Could you check a few things on this model? Use its own coordinates, in mm. Face numbers are marked on the shaded views. A direction names the side the tool comes from. Give positions to 0.01 mm unless a question says otherwise; leave off trailing zeros. Order: outer loops, then holes, each group sorted by start corner. A loop starts at its lowest first (then second) coordinate and runs counter-clockwise, first axis right, second up. Notation, with made-up numbers: (-22, 66) -> (-16, 66) arc R23 ccw to (-16, 99) -> close; hole circle Ø6 at (-36.5, 49). An arc over 180 degrees is marked (long way). Use one line per item in the form item = value. Start each with the question number.
from build123d import *

# Parameters (mm, degrees)
BOSS_EXTRUDE1_DEPTH          = 29
CUT_EXTRUDE1_DEPTH           = 96.799008346
CUT_EXTRUDE2_DEPTH           = 96.799008346
CUT_EXTRUDE2_DEPTH_BACK      = 96.799008346
SKETCH4_W                    = 32.25
SKETCH4_H                    = 6
SKETCH5_W                    = 175.4
SKETCH5_H                    = 34
CUT_EXTRUDE3_DEPTH           = 20.4
SKETCH6_W                    = 29.649504938
SKETCH6_H                    = 34
CUT_EXTRUDE4_DEPTH           = 95.596247283
SKETCH7_W                    = 29.649504938
SKETCH7_H                    = 34
CUT_EXTRUDE5_DEPTH           = 95.596247283
F_5_32_0_14_DIAMETER_HOLE1_D = 3.556
SKETCH13_R                   = 4
CUT_EXTRUDE6_DEPTH           = 106.908356611
FILLET1_R                    = 10
FILLET2_R                    = 10


with BuildPart() as part:
    # Sketch1 → Boss-Extrude1 (new, symmetric)
    with BuildSketch(Plane(origin=(0, 0, 0), x_dir=(1, 0, 0), z_dir=(0, 1, 0))):
        with BuildLine():
            Line((-12.7, 75), (-12.7, -75))
            ThreePointArc((-12.7, -75), (0, -87.7), (12.7, -75))
            Line((12.7, -75), (12.7, 75))
            ThreePointArc((12.7, 75), (0, 87.7), (-12.7, 75))
        make_face()
    extrude(amount=BOSS_EXTRUDE1_DEPTH, both=True)

    # Sketch3 → Cut-Extrude1 (cut, symmetric)
    with BuildSketch(Plane.ZY.offset(12.7)):
        Polygon((-45, 29), (-32.009618943, 21.5), (32.009618943, 21.5), (45, 29), align=None)
    cut_extrude1 = extrude(amount=CUT_EXTRUDE1_DEPTH, both=True, mode=Mode.SUBTRACT)

    # Mirror1: Cut-Extrude1 across plane
    add(cut_extrude1.mirror(Plane.ZX), mode=Mode.SUBTRACT)

    # Sketch4 → Cut-Extrude2 (cut, two sides: drawn at the far end of the back side and taken through both)
    with BuildSketch(Plane.ZY.offset(12.7).offset(-CUT_EXTRUDE2_DEPTH_BACK)):
        with Locations((71.575, 20)):
            Rectangle(SKETCH4_W, SKETCH4_H)
        with Locations((-71.575, 20)):
            Rectangle(SKETCH4_W, SKETCH4_H)
        with Locations((-71.575, -20)):
            Rectangle(SKETCH4_W, SKETCH4_H)
        with Locations((71.575, -20)):
            Rectangle(SKETCH4_W, SKETCH4_H)
    extrude(amount=CUT_EXTRUDE2_DEPTH + CUT_EXTRUDE2_DEPTH_BACK, mode=Mode.SUBTRACT)

    # Sketch5 → Cut-Extrude3 (cut)
    with BuildSketch(Plane.ZY.offset(12.7)):
        Rectangle(SKETCH5_W, SKETCH5_H)
    extrude(amount=-CUT_EXTRUDE3_DEPTH, mode=Mode.SUBTRACT)

    # Sketch6 → Cut-Extrude4 (cut, through all)
    with BuildSketch(Plane.ZY.offset(-7.7)):
        with Locations((70.274752469, 0)):
            Rectangle(SKETCH6_W, SKETCH6_H)
    extrude(amount=-CUT_EXTRUDE4_DEPTH, mode=Mode.SUBTRACT)

    # Sketch7 → Cut-Extrude5 (cut, through all)
    with BuildSketch(Plane.ZY.offset(-7.7)):
        with Locations((-70.274752469, 0)):
            Rectangle(SKETCH7_W, SKETCH7_H)
    extrude(amount=-CUT_EXTRUDE5_DEPTH, mode=Mode.SUBTRACT)

    # 5/32 (0.14) Diameter Hole1 (through all)
    with Locations(Plane(origin=(0, 29, 0), x_dir=(1, 0, 0), z_dir=(0, 1, 0))):
        with Locations((0, -65.221), (-9.779, -75), (9.779, -75), (0, -84.779)):
            f_5_32_0_14_diameter_hole1 = Hole(F_5_32_0_14_DIAMETER_HOLE1_D / 2)

    # Mirror3: 5/32 (0.14) Diameter Hole1 across plane
    add(f_5_32_0_14_diameter_hole1.mirror(Plane.XY), mode=Mode.SUBTRACT)

    # Sketch13 → Cut-Extrude6 (cut, symmetric)
    with BuildSketch(Plane.XZ.offset(29)):
        with Locations(Location((0, -75, 0), (0, 0, 270))):
            Circle(SKETCH13_R)
    cut_extrude6 = extrude(amount=CUT_EXTRUDE6_DEPTH, both=True, mode=Mode.SUBTRACT)

    # Mirror4: Cut-Extrude6 across plane
    add(cut_extrude6.mirror(Plane.XY), mode=Mode.SUBTRACT)

    # Fillet1
    fillet1_edges = [part.edges().sort_by_distance(p)[0] for p in [
        (7.7, 17, 0),
    ]]
    fillet(fillet1_edges, radius=FILLET1_R)

    # Fillet2
    fillet2_edges = [part.edges().sort_by_distance(p)[0] for p in [
        (7.7, -17, 0),
    ]]
    fillet(fillet2_edges, radius=FILLET2_R)


solid = part.part
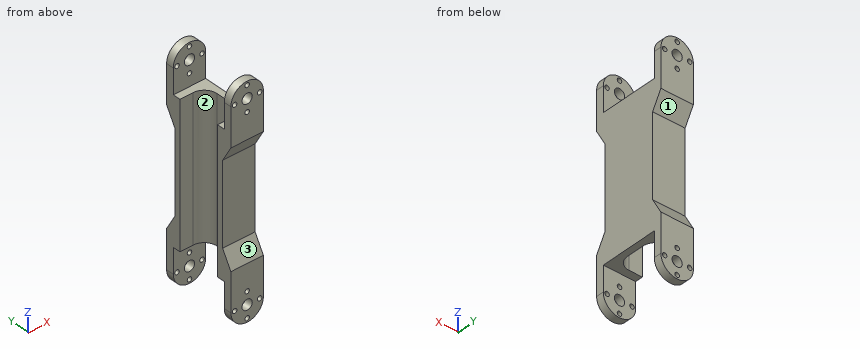
(1) I'm going to push flat-ended pins straight in: pin 1 Ø3 at (x, z) = (0, -65.221) entering from -Y; pin 2 Ø1 at (x, y) = (8, 6) entering from +Z; pin 3 Ø5 at (x, z) = (-5, 32.5) entering from -Y; pin 4 Ø8.5 at (x, z) = (-5, -13.5) entering from +Y. Where does each tip first touch, or does it pass through?
(2) Imagine slicing it at B-B (y = -3.5). Write out the boundary of the cut face in (x, z).
(3) Please list where these lines run through material, in increasing order: probe 1 along X at (y, z) = (-24, 75); probe 2 along Y at (x, z) = (-8.5, -60); probe 3 along Z at (x, y) = (2.5, 25.5).
(4) Imagine slicing it at C-C (z = 29). Write out the boundary of the cut face in (x, y), plus the area to 3 significant figures.
(5) Which directions (+Z, -Z, +X, -X, +Y, -Y) give clear straight access to the entire face, cutting with the end or side of a thin tool? Please do the marked faces 1, 2 and 3.
(6) Imagine slicing it at A-A (z = 47.5). Write out the boundary of the cut face in (x, y).
(7) Imagine slicing it at D-D (x = 10). Give the number of separate pieces and of enclosed holes in the cut face, plus the area to 3 significant figures.
Calculated:
q1.pin_1 = through
q1.pin_2 = 55.45
q1.pin_3 = -23.23
q1.pin_4 = 21.5
q2.outline = (7.7, -55.45) -> (12.7, -55.45) -> (12.7, 55.45) -> (7.7, 55.45) -> close
q3.probe_1 = -12.7 to -11.56, -8 to -4, 4 to 8, 11.56 to 12.7
q3.probe_2 = -29 to -23, 23 to 29
q3.probe_3 = -87.45 to -78.12, -71.88 to -38.94, 38.94 to 71.88, 78.12 to 87.45
q4.outline = (-12.7, -21.5) -> (12.7, -21.5) -> (12.7, 21.5) -> (-12.7, 21.5) -> (-12.7, 17) -> (-2.3, 17) arc R10 cw to (7.7, 7) -> (7.7, -7) arc R10 cw to (-2.3, -17) -> (-12.7, -17) -> close
q4.area = 442 mm2
q5.face_1 = +X, -X, +Y
q5.face_2 = +Z, -Z, -X
q5.face_3 = +X, -X, -Y
q6.outline = (-12.7, -29) -> (12.7, -29) -> (12.7, 29) -> (-12.7, 29) -> (-12.7, 17) -> (-2.3, 17) arc R10 cw to (7.7, 7) -> (7.7, -7) arc R10 cw to (-2.3, -17) -> (-12.7, -17) -> close
q7.separate_pieces = 5
q7.enclosed_holes = 0
q7.area = 5,850 mm2
